```python
from build123d import *

# Parameters (mm, degrees)
F0_R      = 7.272235
F0_R_2    = 6.683406
F1_DEPTH  = 25.4
F2_W      = 22.214184
F2_H      = 111.52488
F3_DEPTH  = 63.5
F5_DEPTH  = 31.140026
F7_DEPTH  = 15.24
F9_DEPTH  = 15.24
F10_R     = 5.88112
F11_DEPTH = 151.526764


with BuildPart() as f1:
    # F0 (on Top) → F1 (new body)
    with BuildSketch(Plane.XY):
        with BuildLine():
            Line((-19.966846, 74.117869), (-19.966846, -75.731389))
            Line((-19.966846, -75.731389), (-19.936258, -75.731389))
            ThreePointArc((-19.936258, -75.731389), (0, -95.667647), (19.936258, -75.731389))
            Line((19.936258, -75.731389), (19.966846, -75.731389))
            Line((19.966846, -75.731389), (19.966846, 74.117869))
            ThreePointArc((19.966846, 74.117869), (0, 95.763324), (-19.966846, 74.117869))
        make_face()
        with Locations((0, -75.731389)):
            Circle(F0_R, mode=Mode.SUBTRACT)
        with Locations((0, 75.731389)):
            Circle(F0_R_2, mode=Mode.SUBTRACT)
    extrude(amount=F1_DEPTH)

    # F2 (on face) → F3 (join)
    with BuildSketch(Plane.XY.offset(25.4)):
        Rectangle(F2_W, F2_H)
    extrude(amount=F3_DEPTH)

    # F4 (on face) → F5 (cut, through all)
    with BuildSketch(Plane.YZ.offset(11.107092)):
        with BuildLine():
            Line((40.165234, 88.9), (-40.165234, 88.9))
            ThreePointArc((-40.165234, 88.9), (0, 48.734766), (40.165234, 88.9))
        make_face()
    extrude(amount=-F5_DEPTH, mode=Mode.SUBTRACT)

    # F6 (on face) → F7 (join)
    with BuildSketch(Plane.XZ.offset(55.76244)):
        with BuildLine():
            Line((5.916213, 88.9), (11.107092, 88.9))
            ThreePointArc((11.107092, 88.9), (0, 100.007092), (-11.107092, 88.9))
            Line((-11.107092, 88.9), (-5.916213, 88.9))
            ThreePointArc((-5.916213, 88.9), (0, 94.816213), (5.916213, 88.9))
        make_face()
    extrude(amount=-F7_DEPTH)

    # F8 (on face) → F9 (join)
    with BuildSketch(Plane(origin=(0, 55.76244, 0), x_dir=(-1, 0, 0), z_dir=(0, 1, 0))):
        with BuildLine():
            Line((-11.068059, 88.9), (11.068059, 88.9))
            ThreePointArc((11.068059, 88.9), (0, 99.968059), (-11.068059, 88.9))
        make_face()
    extrude(amount=-F9_DEPTH)

    # F10 (on face) → F11 (cut, through all)
    with BuildSketch(Plane.XZ.offset(55.76244)):
        with Locations((0, 88.9)):
            Circle(F10_R)
    extrude(amount=-F11_DEPTH, mode=Mode.SUBTRACT)


solid = f1.part
```
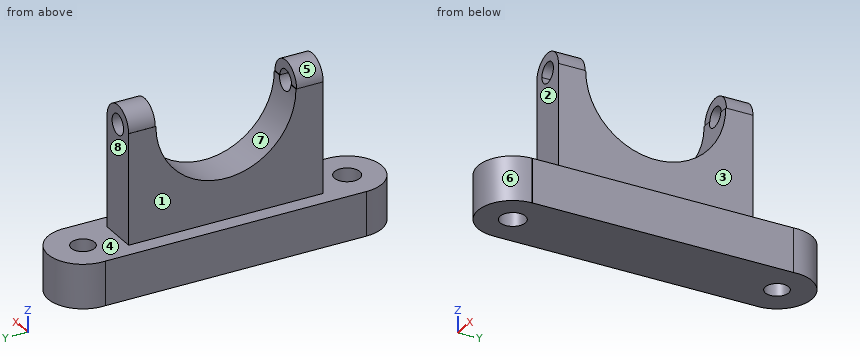
Geometry check sheet. Reference: the model listing, model coordinates, mm. Face numbers are marked on the shaded views. A direction names the side the tool comes from. Coordinates: 2 decimals unless noted, no trailing zeros. Write each loop counter-clockwise with the first axis right and the second up, starting at its lowest first coordinate (ties: lowest second). Pieces come first, ordered by that corner, then holes. Notation, with made-up numbers: M 35,-37.5 L 73,-37.5 A20 ccw 73,-1.5 Z; hole C -5,-13 d7. An arc over 180 degrees is marked long. Use one line per item in the form item = value. Start each with the question number.
1) Set-up check for the marked faces 1, 2, 3 and 4: record each of +Z, -Z, +X, -X, +Y, -Y from which the full face is reachable in a straight line by a thin tool's end or side.
2) Release check for a two-part mould opening along Y. For the marked faces 5, 6, 7 and 8 record: pulls with the +Y half, pulls with the -Y half, needs draft (parallel to the pull), parting line crosses it, or undercut.
3) Section check C-C on z = 60.5. Enter the section's corners in (x, y).
4) Section check A-A on x = 0. Enter the section's corners in (y, z).
5) Section check D-D on y = 0. Enter the section's corners in (x, z), and give its area (3 significant figures).
6) Go/stop test with flat-tipped pins: pin 1 Ø2.5 at (x, y) = (8, 47.5) entering from +Z; pin 2 Ø11 at (x, z) = (-4, 66) entering from -Y; pin 3 Ø7.5 at (y, z) = (-4.5, 16) entering from +X; pin 4 Ø1.5 at (x, y) = (-9.5, 71.5) entering from -Z. Record where each tip stops, or that it passes through.
7) Thickness scan on probe 1 along Y at (x, z) = (0, 20.25); probe 2 along X at (y, z) = (76, 18); probe 3 along Y at (x, z) = (1, 7). Record the ranges inside material, lowest first. Write a range as from..to.
Responses:
q1.face_1 = +Z, -X, +Y, -Y
q1.face_2 = +Z, +X, -X, -Y
q1.face_3 = +Z, +X, +Y, -Y
q1.face_4 = +Z
q2.face_5 = needs draft
q2.face_6 = pulls with the -Y half
q2.face_7 = undercut
q2.face_8 = pulls with the +Y half
q3.outline = M -11.11,-55.76 L 11.11,-55.76 L 11.11,-28.4 L -11.11,-28.4 Z; M -11.11,28.4 L 11.11,28.4 L 11.11,55.76 L -11.11,55.76 Z
q4.outline = M -95.67,0 L -83,0 L -83,25.4 L -95.67,25.4 Z; M -68.46,0 L 69.05,0 L 69.05,25.4 L 55.76,25.4 L 55.76,83.02 L 39.73,83.02 A40.17 cw -39.73,83.02 L -55.76,83.02 L -55.76,25.4 L -68.46,25.4 Z; M -55.76,94.82 L -40.52,94.82 L -40.52,100.01 L -55.76,100.01 Z; M 40.52,94.78 L 55.76,94.78 L 55.76,99.97 L 40.52,99.97 Z; M 82.41,0 L 95.76,0 L 95.76,25.4 L 82.41,25.4 Z
q5.outline = M -19.97,0 L 19.97,0 L 19.97,25.4 L 11.11,25.4 L 11.11,48.73 L -11.11,48.73 L -11.11,25.4 L -19.97,25.4 Z
q5.area = 1,530 mm2
q6.pin_1 = 97.67
q6.pin_2 = -55.76
q6.pin_3 = 19.97
q6.pin_4 = 0
q7.probe_1 = -95.67..-83, -68.46..69.05, 82.41..95.76
q7.probe_2 = -20.03..-6.68, 6.68..20.03
q7.probe_3 = -95.64..-82.93, -68.53..69.12, 82.34..95.74
